Could you check a few things on this model? Use its own coordinates, in mm. A direction names the side the tool comes from. Give positions to 0.01 mm unless a question says otherwise; leave off trailing zeros. Loops run counter-clockwise (first coordinate to the right, second up) from the corner with the lowest first, then second, coordinate; pieces in that order, holes last. Notation, with made-up numbers: (3, 34) - (34, 34) arc R17 ccw to (34, 50) - close; hole circle Ø11 at (-38, 66.5). An arc over 180 degrees is marked (long way). One line per item, written item: value. Start each with the question number.
Q1. For faces 1 (the face through (13.155, -4.008, 0.479)), 2 (the face through (8, 2, 0)), which set-ups out of +Z, -Z, +X, -X, +Y, -Y let a thin tool reach every point of the face, with its end or its side?
Q2. I'm going to push flat-ended pins straight in: P1, Ø8, axis at x = 14.5, y = -9, coming from the -Z side (3 decimals); P2, Ø3, axis at x = 7, y = 16.5, coming from the -Z side; P3, Ø6, axis at y = -1.5, z = -26, coming from the +X side; P4, Ø1.5, axis at x = 12, z = 0, coming from the +Y side. Where does each tip first touch, or does it pass through?
Q3. If I drill on line 1 (Z direction, x = 12.5, y = 0); line 2 (X direction, y = 27.5, z = -10.5); line 3 (Z direction, x = 5.25, y = -0.5), over which ranges is the centre line in solid material (lowest first)? Write a range as from..to.
Q4. I want a section at A-A (z = 0). Please give me the cut outline in (x, y) (3 decimals).
Q5. I want a section at D-D (x = 6.5). Please give me the cut outline in (y, z).
Q6. If we mould it in two halves opening along Y, with no side actions, what happens to faces 3 (the face through (2.465, 11.908, 20.548)), 4 (the face through (2.54, -9.05, 33.81)), 5 (the face through (2.46, 4.07, -29.44)), 6 (the face through (5, -8, 0))? For each: released by +Y, released by -Y, zero draft, split by the parting line, or undercut.
Q7. I want a section at C-C (y = 1). Please give me the cut outline in (x, z), then the cut area to 3 significant figures.
Q8. I want a section at B-B (x = 12). Please give me the cut outline in (y, z) (3 decimals), then the cut area to 3 significant figures.
```python
from build123d import *

# Parameters (mm, degrees)
BASPROSKE_W                     = 5
BASPROSKE_H                     = 35
TOOTHCUT_DEPTH                  = 50.749371855
TEETHCUTS_COUNT                 = 12
TEETHCUTS_ANGLE                 = 330
BORSKE_R                        = 0.4
BORE_DEPTH                      = 50.0000508
SKETCH1_R                       = 2
CUT_EXTRUDE1_DEPTH              = 49.388618122
SKETCH2_R                       = 2
BOSS_EXTRUDE1_DEPTH             = 11
M3X0_5_TAPPED_HOLE1_D           = 2.5
M3X0_5_TAPPED_HOLE1_DEPTH       = 7.5
M3X0_5_TAPPED_HOLE1_CSINK_D     = 3.45
M3X0_5_TAPPED_HOLE1_CSINK_ANGLE = 90
M3X0_5_TAPPED_HOLE1_TIP         = 0.751075774


with BuildPart() as part:
    # BasProSke → Base-Revolve (revolve)
    with BuildSketch(Plane(origin=(0, 0, 0), x_dir=(1, 0, 0), z_dir=(0, 1, 0)), mode=Mode.PRIVATE) as base_revolve_sk:
        with Locations((2.5, 17.5)):
            Rectangle(BASPROSKE_W, BASPROSKE_H)
    revolve(base_revolve_sk.sketch.rotate(Axis((-10, 0, 0), (1, 0, 0)), 180), axis=Axis((-10, 0, 0), (1, 0, 0)))

    # TooCutSke → ToothCut (cut, through all)
    with BuildSketch(Plane(origin=(0, 0, 0), x_dir=(0, 0, -1), z_dir=(1, 0, 0))):
        with BuildLine():
            ThreePointArc((2.779025365, 23.585843615), (0, 23.749), (-2.779025365, 23.585843615))
            ThreePointArc((-2.779025365, 23.585843615), (-4.116196739, 29.530367698), (-8.200466404, 34.051886819))
            ThreePointArc((-8.200466404, 34.051886819), (0, 35.0254), (8.200466404, 34.051886819))
            ThreePointArc((8.200466404, 34.051886819), (4.116196739, 29.530367698), (2.779025365, 23.585843615))
        make_face()
    toothcut = extrude(amount=TOOTHCUT_DEPTH, mode=Mode.SUBTRACT)

    # TeethCuts: ToothCut ×12 about axis
    teethcuts_axis = Axis((-10, 0, 0), (1, 0, 0))
    for i in range(1, TEETHCUTS_COUNT):
        add(toothcut.rotate(teethcuts_axis, i * TEETHCUTS_ANGLE / (TEETHCUTS_COUNT - 1)), mode=Mode.SUBTRACT)

    # BorSke → Bore (cut, symmetric)
    with BuildSketch(Plane(origin=(0, 0, 0), x_dir=(0, 0, -1), z_dir=(1, 0, 0))):
        with Locations(Location((0, 0, 0), (0, 0, 180))):
            Circle(BORSKE_R)
    extrude(amount=BORE_DEPTH, both=True, mode=Mode.SUBTRACT)

    # Sketch1 → Cut-Extrude1 (cut, through all)
    with BuildSketch(Plane(origin=(5, 0, 0), x_dir=(0, 0, -1), z_dir=(1, 0, 0))):
        Circle(SKETCH1_R)
    extrude(amount=-CUT_EXTRUDE1_DEPTH, mode=Mode.SUBTRACT)

    # Sketch2 → Boss-Extrude1 (add)
    with BuildSketch(Plane.ZY.offset(-5)):
        with BuildLine():
            Line((-3.872983346, -7), (3.872983346, -7))
            ThreePointArc((3.872983346, -7), (6.891439137, -4.063012013), (8, 0))
            ThreePointArc((8, 0), (-4.063012013, 6.891439137), (-3.872983346, -7))
        make_face()
        with Locations(Location((0, 0, 0), (0, 0, 180))):
            Circle(SKETCH2_R, mode=Mode.SUBTRACT)
    extrude(amount=-BOSS_EXTRUDE1_DEPTH)

    # M3x0.5 Tapped Hole1
    with Locations(Plane(origin=(0, -7, 0), x_dir=(-1, 0, 0), z_dir=(0, -1, 0))):
        with Locations((-12, 0)):
            CounterSinkHole(M3X0_5_TAPPED_HOLE1_D / 2, M3X0_5_TAPPED_HOLE1_CSINK_D / 2, depth=M3X0_5_TAPPED_HOLE1_DEPTH, counter_sink_angle=M3X0_5_TAPPED_HOLE1_CSINK_ANGLE)
            with Locations((0, 0, -(M3X0_5_TAPPED_HOLE1_DEPTH + M3X0_5_TAPPED_HOLE1_TIP / 2))):  # 118° drill point
                Cone(0, M3X0_5_TAPPED_HOLE1_D / 2, M3X0_5_TAPPED_HOLE1_TIP, mode=Mode.SUBTRACT)


solid = part.part
```
Worked answers:
1. face 1: -Y
1. face 2: +X, -X
2. P1: stops at z = -6.245
2. P2: passes through
2. P3: stops at x = 5
2. P4: stops at y = 8
3. line 1: z = -8..-2, 2..8
3. line 2: x = 0..5
3. line 3: z = -7.98..-1.94, 1.94..7.98
4. outline: (0, -23.749) - (5, -23.749) - (5, -7) - (10.275, -7) - (10.75, -6.525) - (10.75, -2) - (0, -2) - close; (0, 2) - (16, 2) - (16, 8) - (5, 8) - (5, 23.749) - (0, 23.749) - close; (13.25, -6.525) - (13.725, -7) - (16, -7) - (16, -2) - (13.25, -2) - close
5. outline: (-7, -3.87) arc R8 ccw (long way) to (-7, 3.87) - close; hole circle Ø4 at (0, 0)
6. face 3: undercut
6. face 4: released by -Y
6. face 5: undercut
6. face 6: zero draft
7. outline: (0, -23.73) - (5, -23.73) - (5, -7.94) - (16, -7.94) - (16, -1.73) - (0, -1.73) - close; (0, 1.73) - (16, 1.73) - (16, 7.94) - (5, 7.94) - (5, 23.73) - (0, 23.73) - close
7. area: 356 mm²
8. outline: (-7, -3.873) arc R8 ccw (long way) to (-7, 3.873) - (-7, 1.725) - (-6.525, 1.25) - (-1.561, 1.25) arc R2 cw (long way) to (-1.561, -1.25) - (-6.525, -1.25) - (-7, -1.725) - close
8. area: 170 mm²
